Verification items for the finished model (mm, model axes). A direction names the side the tool comes from. Coordinates: 2 decimals unless noted, no trailing zeros. Write each loop counter-clockwise with the first axis right and the second up, starting at its lowest first coordinate (ties: lowest second). Pieces come first, ordered by that corner, then holes. Notation, with made-up numbers: (44, 81.5) -> (86, 81.5) arc R20 cw to (86, 85.5) -> close; hole circle Ø4 at (22.25, 47). An arc over 180 degrees is marked (long way). Answer in a Markdown table with one row per item.
```python
from build123d import *

# Parameters (mm, degrees)
SKETCH1_W                      = 76.2
SKETCH1_H                      = 190.5
BASE_FLANGE1_DEPTH             = 3.2639
EDGE_FLANGE1_STRIP_W           = 15.5956
EDGE_FLANGE1_STRIP_H           = 3.2639
EDGE_FLANGE1_STRIP_CUT_DEPTH   = 190.5
EDGE_FLANGE1_STRIP_2_W         = 15.5956
EDGE_FLANGE1_STRIP_2_H         = 3.2639
EDGE_FLANGE1_STRIP_CUT_2_DEPTH = 190.5
EDGE_FLANGE1_DEPTH             = 190.5
EDGE_FLANGE1_BEND_DEPTH        = 190.5
F_10_0_1935_DIAMETER_HOLE1_D   = 4.9149
F_10_0_1935_DIAMETER_HOLE2_D   = 4.9149
CUT_EXTRUDE1_DEPTH             = 125.595997127
FILLET2_R                      = 6.35


# Sheet-metal steps are written as plain solids
with BuildPart() as part:
    # Sketch1 → Base-Flange1 (new body)
    with BuildSketch(Plane(origin=(0, 0, 0), x_dir=(1, 0, 0), z_dir=(0, 1, 0))):
        Rectangle(SKETCH1_W, SKETCH1_H)
    extrude(amount=-BASE_FLANGE1_DEPTH)

    # Edge-Flange1 strip (across the edge) → Edge-Flange1 strip cut (cut)
    with BuildSketch(Plane(origin=(38.1, -3.2639, -95.25), x_dir=(-1, 0, 0), z_dir=(0, 0, 1))):
        with Locations((-3.2639, -1.63195)):
            Rectangle(EDGE_FLANGE1_STRIP_W, EDGE_FLANGE1_STRIP_H)
    extrude(amount=EDGE_FLANGE1_STRIP_CUT_DEPTH, mode=Mode.SUBTRACT)

    # Edge-Flange1 strip 2 (across the edge) → Edge-Flange1 strip cut 2 (cut)
    with BuildSketch(Plane(origin=(-38.1, -3.2639, 95.25), x_dir=(1, 0, 0), z_dir=(0, 0, -1))):
        with Locations((-3.2639, -1.63195)):
            Rectangle(EDGE_FLANGE1_STRIP_2_W, EDGE_FLANGE1_STRIP_2_H)
    extrude(amount=EDGE_FLANGE1_STRIP_CUT_2_DEPTH, mode=Mode.SUBTRACT)

    # Edge-Flange1 section (across the edge) → Edge-Flange1 (add)
    with BuildSketch(Plane(origin=(38.1, -3.2639, -95.25), x_dir=(-1, 0, 0), z_dir=(0, 0, 1))):
        with BuildLine():
            Line((0, 1.27), (0, 22.1361))
            Line((0, 22.1361), (3.2639, 22.1361))
            Line((3.2639, 22.1361), (3.2639, 1.27))
            ThreePointArc((3.2639, 1.27), (3.635874388, 0.371974388), (4.5339, 0))
            Line((4.5339, 0), (4.5339, -3.2639))
            ThreePointArc((4.5339, -3.2639), (1.327948565, -1.935951435), (0, 1.27))
        make_face()
    extrude(amount=EDGE_FLANGE1_DEPTH)

    # Edge-Flange1 section 2 (across the edge) → Edge-Flange1 bend (add)
    with BuildSketch(Plane(origin=(-38.1, -3.2639, 95.25), x_dir=(1, 0, 0), z_dir=(0, 0, -1))):
        with BuildLine():
            Line((0, 1.27), (0, 22.1361))
            Line((0, 22.1361), (3.2639, 22.1361))
            Line((3.2639, 22.1361), (3.2639, 1.27))
            ThreePointArc((3.2639, 1.27), (3.635874388, 0.371974388), (4.5339, 0))
            Line((4.5339, 0), (4.5339, -3.2639))
            ThreePointArc((4.5339, -3.2639), (1.327948565, -1.935951435), (0, 1.27))
        make_face()
    extrude(amount=EDGE_FLANGE1_BEND_DEPTH)

    # #10 (0.1935) Diameter Hole1 (through all)
    with Locations(Plane(origin=(0, 0, 0), x_dir=(1, 0, 0), z_dir=(0, 1, 0))):
        with Locations((-25.4, 82.55), (25.4, 82.55), (-25.4, 0), (25.4, 0), (25.4, -82.55), (-25.4, -82.55)):
            Hole(F_10_0_1935_DIAMETER_HOLE1_D / 2)

    # #10 (0.1935) Diameter Hole2 (through all)
    with Locations(Plane(origin=(38.1, 0, 0), x_dir=(0, 0, -1), z_dir=(1, 0, 0))):
        with Locations((-63.5, -14.2875), (63.5, -14.2875)):
            Hole(F_10_0_1935_DIAMETER_HOLE2_D / 2)

    # Sketch19 → Cut-Extrude1 (cut, through all)
    with BuildSketch(Plane(origin=(38.1, 0, 0), x_dir=(0, 0, -1), z_dir=(1, 0, 0))):
        Polygon((-95.25, -9.525), (-63.5, -25.4), (-95.25, -25.4), align=None)
        Polygon((63.5, -25.4), (95.25, -25.4), (95.25, -9.525), align=None)
    extrude(amount=-CUT_EXTRUDE1_DEPTH, mode=Mode.SUBTRACT)

    # Fillet2
    fillet2_edges = [part.edges().sort_by_distance(p)[0] for p in [
        (36.46805, -25.4, 63.5),
        (36.46805, -9.525, 95.25),
        (-36.46805, -9.525, 95.25),
        (-36.46805, -25.4, 63.5),
        (36.46805, -25.4, -63.5),
        (36.46805, -9.525, -95.25),
        (-36.46805, -25.4, -63.5),
        (-36.46805, -9.525, -95.25),
    ]]
    fillet(fillet2_edges, radius=FILLET2_R)


solid = part.part
```
1. Go/stop test with flat-tipped pins: pin 1 (8 mm diameter, centred on x = -25.4, z = 0, fed in from -Y); pin 2 (1.5 mm diameter, centred on y = -3, z = -74.5, fed in from -X). Record where each tip stops, or that it passes through.
Findings below:
| item | result |
|---|---|
| pin 1 | stops at y = -3.26 |
| pin 2 | stops at x = -38.03 |
2. Material ranges on probe 1 along Z at (x, y) = (-25.4, -1.6); probe 2 along X at (y, z) = (-13.75, -59); probe 3 along Y at (x, z) = (-21, -20.5), recorded low to high. Write a range as from..to.
Findings below:
| item | result |
|---|---|
| probe 1 | z = -95.25..-85.01, -80.09..-2.46, 2.46..80.09, 85.01..95.25 |
| probe 2 | x = -38.1..-34.84, 34.84..38.1 |
| probe 3 | y = -3.26..0 |
3. Sectioned sample at D-D, the plane z = 25.5. Record the cut outline in (x, y), and give its area (3 significant figures).
Findings below:
| item | result |
|---|---|
| outline | (-38.1, -25.4) -> (-34.84, -25.4) -> (-34.84, -4.53) arc R1.27 cw to (-33.57, -3.26) -> (33.57, -3.26) arc R1.27 cw to (34.84, -4.53) -> (34.84, -25.4) -> (38.1, -25.4) -> (38.1, -4.53) arc R4.53 ccw to (33.57, 0) -> (-33.57, 0) arc R4.53 ccw to (-38.1, -4.53) -> close |
| area | 385 mm² |
4. Sectioned sample at C-C, the plane z = -82.55. Record the cut outline in (x, y) (3 decimals).
Findings below:
| item | result |
|---|---|
| outline | (-38.1, -15.875) -> (-34.836, -15.875) -> (-34.836, -4.534) arc R1.27 cw to (-33.566, -3.264) -> (-27.857, -3.264) -> (-27.857, 0) -> (-33.566, 0) arc R4.534 ccw to (-38.1, -4.534) -> close; (-22.943, -3.264) -> (22.943, -3.264) -> (22.943, 0) -> (-22.943, 0) -> close; (27.857, -3.264) -> (33.566, -3.264) arc R1.27 cw to (34.836, -4.534) -> (34.836, -15.875) -> (38.1, -15.875) -> (38.1, -4.534) arc R4.534 ccw to (33.566, 0) -> (27.857, 0) -> close |
5. Release check for a two-part mould opening along Y. For faces 1 (the face through (-36.49, -15.78, 61.55)), 2 (the face through (0, 0, -1)), 3 (the face through (0, -3.264, -1)), 4 (the face through (27.855, -1.655, -0.108)) record: released by +Y, released by -Y, zero draft, split by the parting line, or undercut.
Findings below:
| item | result |
|---|---|
| face 1 | undercut |
| face 2 | released by +Y |
| face 3 | released by -Y |
| face 4 | zero draft |
6. Access from +Z, -Z, +X, -X, +Y, -Y to the whole of each face (thin tool, end or side, straight path). Record for faces 5 (the face through (-36.491, -8.897, 94.327)), 6 (the face through (-34.836, -15, 1)).
Findings below:
| item | result |
|---|---|
| face 5 | +Z, +X, -X, -Y |
| face 6 | +Z, -Z, -Y |
7. Sectioned sample at B-B, the plane y = -20.25. Record the cut outline in (x, z).
Findings below:
| item | result |
|---|---|
| outline | (-38.1, -73.8) -> (-34.84, -73.8) -> (-34.84, 73.8) -> (-38.1, 73.8) -> close; (34.84, -73.8) -> (38.1, -73.8) -> (38.1, 73.8) -> (34.84, 73.8) -> close |
8. Sectioned sample at A-A, the plane x = 25.4. Record the cut outline in (y, z).
Findings below:
| item | result |
|---|---|
| outline | (-3.26, -95.25) -> (0, -95.25) -> (0, -85.01) -> (-3.26, -85.01) -> close; (-3.26, -80.09) -> (0, -80.09) -> (0, -2.46) -> (-3.26, -2.46) -> close; (-3.26, 2.46) -> (0, 2.46) -> (0, 80.09) -> (-3.26, 80.09) -> close; (-3.26, 85.01) -> (0, 85.01) -> (0, 95.25) -> (-3.26, 95.25) -> close |
